```python
from build123d import *

# Parameters (mm, degrees)
SKETCH1_R             = 3.5
BASE_EXTRUDE_DEPTH    = 3.4
RBODY_SKETCH_R        = 5.55
RBODY_DEPTH           = 9.6
ELBOW_ANGLE           = 90
SKETCH3_R             = 3.5
BOSS_EXTRUDE1_DEPTH   = 6.6
BOSS_EXTRUDE2_DEPTH   = 0.9
NUT_DEPTH             = 5.4
THREADS_SKETCH_W      = 2.415
THREADS_SKETCH_H      = 4
THREAD_CHAMFER_SIZE   = 0.25
RTUBE_START           = -13.3
RTUBE_SKETCH_R        = 3.175
RTUBE_DEPTH           = 13.3
RTUBE_RADIUS_R        = 0.5
DIAMETER_R            = 1.25
SKETCH4_W             = 3.5
SKETCH4_H             = 0.55
PORT_THREADS_REACH    = 29.062
PORT_THREADS_SKETCH_R = 1.25


with BuildPart() as part:
    # Sketch1 → Base-Extrude (new body)
    with BuildSketch(Plane(origin=(0, 0, 0), x_dir=(0, 0, -1), z_dir=(1, 0, 0))):
        Circle(SKETCH1_R)
    extrude(amount=BASE_EXTRUDE_DEPTH)

    # RBody_Sketch → RBody (add)
    with BuildSketch(Plane(origin=(3.4, 0, 0), x_dir=(0, 0, -1), z_dir=(1, 0, 0))):
        Circle(RBODY_SKETCH_R)
    extrude(amount=RBODY_DEPTH)

    # RBody_Chamfer: read off the stored shape, not the designer's step
    # RBody_Chamfer outline → RBody_Chamfer (revolve, cut)
    with BuildSketch(Plane.YX):
        Polygon((5.55, 4.14613898), (3.5, 3.4), (5.55, 3.4), align=None)
    revolve(axis=Axis((0, 0, 0), (1, 0, 0)), mode=Mode.SUBTRACT)

    # RRelease_Sketch → RRelease (revolve)
    with BuildSketch(Plane.XY, mode=Mode.PRIVATE) as rrelease_sk:
        with BuildLine():
            Line((13, 3.925), (13.9, 3.925))
            Line((13.9, 3.925), (13.9, 5.025))
            Line((13.9, 5.025), (14.9, 5.025))
            ThreePointArc((14.9, 5.025), (15.253553391, 4.878553391), (15.4, 4.525))
            Line((15.4, 4.525), (15.4, 0))
            Line((15.4, 0), (13, 0))
            Line((13, 0), (13, 3.925))
        make_face()
    revolve(rrelease_sk.sketch.rotate(Axis((12.597722381, 0, 0), (1, 0, 0)), 90), axis=Axis((12.597722381, 0, 0), (1, 0, 0)))

    # Elbow_Sketch → Elbow (revolve)
    with BuildSketch(Plane.ZY):
        with BuildLine():
            Line((-3.5, 0), (3.5, 0))
            ThreePointArc((3.5, 0), (0, 3.5), (-3.5, 0))
        make_face()
    revolve(axis=Axis((0, 0, -6.487672297), (0, 0, 1)), revolution_arc=ELBOW_ANGLE)

    # Sketch3 → Boss-Extrude1 (add)
    with BuildSketch(Plane.XZ):
        with Locations(Location((0, 0, 0), (0, 0, 90))):
            Circle(SKETCH3_R)
    extrude(amount=BOSS_EXTRUDE1_DEPTH)

    # Sketch8 → Boss-Extrude2 (add, symmetric)
    with BuildSketch(Plane.XY):
        with BuildLine():
            Line((-3.5, -6.6), (-3.5, 3.75))
            ThreePointArc((-3.5, 3.75), (-3.207106781, 4.457106781), (-2.5, 4.75))
            Line((-2.5, 4.75), (4.14613898, 4.75))
            Line((4.14613898, 4.75), (4.14613898, 0))
            Line((4.14613898, 0), (0, 0))
            Line((0, 0), (0, -6.6))
            Line((0, -6.6), (-3.5, -6.6))
        make_face()
    extrude(amount=BOSS_EXTRUDE2_DEPTH, both=True)

    # Nut_Sketch → Nut (add)
    with BuildSketch(Plane(origin=(0, -12, 0), x_dir=(-1, 0, 0), z_dir=(0, 1, 0))):
        Polygon((4.041451884, 0), (2.020725942, 3.5), (-2.020725942, 3.5), (-4.041451884, 0), (-2.020725942, -3.5), (2.020725942, -3.5), align=None)
    extrude(amount=NUT_DEPTH)

    # Nut_Chamfer_Sketch → Nut_Chamfer (revolve, cut)
    with BuildSketch(Plane.XY):
        Polygon((-3.5, -6.6), (-4.041451884, -6.6), (-4.041451884, -6.912607391), align=None)
        Polygon((-4.041451884, -11.687392609), (-3.5, -12), (-4.041451884, -12), align=None)
    revolve(axis=Axis((0, -1.551633987, 0), (0, 1, 0)), mode=Mode.SUBTRACT)

    # Threads_Sketch → Threads (revolve)
    with BuildSketch(Plane.XY):
        with Locations((-1.2075, -14)):
            Rectangle(THREADS_SKETCH_W, THREADS_SKETCH_H)
    revolve(axis=Axis((0, 0, 0), (0, -1, 0)))

    # Thread_Chamfer
    thread_chamfer_edges = [part.edges().sort_by_distance(p)[0] for p in [
        (2.415, -16, 0),
    ]]
    chamfer(thread_chamfer_edges, length=THREAD_CHAMFER_SIZE)

    # RTube_Sketch → RTube (cut)
    with BuildSketch(Plane(origin=(15.4, 0, 0), x_dir=(0, 0, -1), z_dir=(1, 0, 0)).offset(RTUBE_START)):
        Circle(RTUBE_SKETCH_R)
    extrude(amount=RTUBE_DEPTH, mode=Mode.SUBTRACT)

    # RTube_Radius
    rtube_radius_edges = [part.edges().sort_by_distance(p)[0] for p in [
        (15.4, 0, 3.175),
    ]]
    fillet(rtube_radius_edges, radius=RTUBE_RADIUS_R)

    # Port_Curve: sweep along a path in Profile
    with BuildLine(Plane.XY) as port_curve_path:
        ThreePointArc((2.1, 0), (0.61507576, -0.61507576), (0, -2.1))
    # Diameter → Port_Curve (sweep, cut)
    with BuildSketch(Plane(origin=(2.1, 0, 0), x_dir=(0, 0, -1), z_dir=(1, 0, 0))):
        Circle(DIAMETER_R)
    sweep(path=port_curve_path.line, mode=Mode.SUBTRACT)

    # Sketch4 → Revolve1 (revolve)
    with BuildSketch(Plane.XY, mode=Mode.PRIVATE) as revolve1_sk:
        with Locations((-1.75, -12.275)):
            Rectangle(SKETCH4_W, SKETCH4_H)
    revolve(revolve1_sk.sketch.rotate(Axis((0, 0, 0), (0, -1, 0)), 180), axis=Axis((0, 0, 0), (0, -1, 0)))

    # Port_Threads_Sketch → Port_Threads (cut, up to next)
    with BuildSketch(Plane(origin=(0, -16, 0), x_dir=(-1, 0, 0), z_dir=(0, 1, 0)), mode=Mode.PRIVATE) as port_threads_sk1:
        Circle(PORT_THREADS_SKETCH_R)
    port_threads_tool1 = extrude(port_threads_sk1.sketch, amount=PORT_THREADS_REACH, mode=Mode.PRIVATE) & part.part
    add(port_threads_tool1.solids().sort_by_distance((0, -16, 0))[0], mode=Mode.SUBTRACT)


solid = part.part
```
Verification items for the finished model (mm, model axes). A direction names the side the tool comes from. Round coordinates to 2 decimals unless told otherwise and drop trailing zeros. Write each loop counter-clockwise with the first axis right and the second up, starting at its lowest first coordinate (ties: lowest second). Pieces come first, ordered by that corner, then holes. Notation, with made-up numbers: (60.5, 84) - (95.5, 84) arc R18 cw to (95.5, 112) - close; hole circle Ø5 at (-25.75, 69). An arc over 180 degrees is marked (long way). Answer as a JSON object with one key per item and string values. Group by question number.
Q1. Thickness scan on line 1 (Z direction, x = 0, y = -6.5); line 2 (Y direction, x = 11.25, z = 0) (3 decimals); line 3 (X direction, y = -3.75, z = -3). Record the ranges inside material, lowest first.
Q2. Section check C-C, the plane y = -13. Enter the section's corners in (x, z) (3 decimals).
Q3. Mould release check, pull along Y, two halves, no side actions. Record for faces 1 (the conical face through (3.69, -6.71, 0.01)), 2 (the cylindrical face through (14.41, -0.22, -5.02)), 3 (the flat face through (15.4, -4, 0)), 4 (the conical face through (-1.8, -11.9, -3.2)): released by +Y, released by -Y, zero draft, split by the parting line, or undercut.
Q4. Section check B-B, the plane x = 9.25. Enter the section's corners in (y, z) (3 decimals).
Q5. Go/stop test with flat-tipped pins: pin 1 Ø5 at (y, z) = (3, -1) entering from -X; pin 2 Ø6 at (x, y) = (2, 0.5) entering from +Z; pin 3 Ø1.9 at (y, z) = (-0.5, -0.5) entering from +X; pin 4 Ø6 at (x, z) = (9, -0.5) entering from -Y. Record where each tip stops, or that it passes through.
Q6. Tool access check on faces 5 (the cylindrical face through (1.676, 0.916, -3.378)), 6 (the flat face through (1, 4.75, 0)), 7 (the flat face through (-1, 4, -0.9)). Record the directions out of +Z, -Z, +X, -X, +Y, -Y that give a thin tool (end or side, any length) a straight path to the whole face; none if there is none.
Q7. Section check A-A, the plane y = -8. Enter the section's corners in (x, z), plus the area to 3 significant figures.
Found:
{
 "1": {"line 1": "z = -3.5 to -1.25, 1.25 to 3.5", "line 2": "y = -5.55 to -3.175, 3.175 to 5.55", "line 3": "x = -1.8 to 1.8, 3.87 to 13, 13.9 to 15.32"},
 "2": {"outline": "circle Ø4.83 at (0, 0); hole circle Ø2.5 at (0, 0)"},
 "3": {"face 1": "undercut", "face 2": "split by the parting line", "face 3": "zero draft", "face 4": "released by -Y"},
 "4": {"outline": "circle Ø11.1 at (0, 0); hole circle Ø6.35 at (0, 0)"},
 "5": {"pin 1": "stops at x = -3.5", "pin 2": "stops at z = 5.55", "pin 3": "stops at x = 2.1", "pin 4": "stops at y = -5.55"},
 "6": {"face 5": "-Z", "face 6": "+Z, -Z, -X, +Y", "face 7": "-Z, -X, +Y"},
 "7": {"outline": "(-4.04, 0) - (-2.02, -3.5) - (2.02, -3.5) - (4.04, 0) - (2.02, 3.5) - (-2.02, 3.5) - close; hole circle Ø2.5 at (0, 0)", "area": "37.5 mm^2"}
}
